Geometry: final body of the model. Coordinates: model frame, mm. A direction names the side the tool comes from. Give positions to 0.01 mm unless a question says otherwise; leave off trailing zeros. Write each loop counter-clockwise with the first axis right and the second up, starting at its lowest first coordinate (ties: lowest second). Pieces come first, ordered by that corner, then holes. Notation, with made-up numbers: M 2.5,70 L 20.5,70 A25 cw 20.5,104 Z; hole C 78.25,-37 d6. An arc over 180 degrees is marked long. Answer as a JSON object with one key per item and string values.
from build123d import *
from build123d.topology import SkipClean

# Parameters (mm, degrees)
SKETCH_1_R          = 3.25
EXTRUDE_1_DEPTH     = 29
CUT_EXTRUDE_START   = -5
SKETCH_2_OUTSIDE_W  = 14.584
SKETCH_2_OUTSIDE_H  = 14.584
SKETCH_2_OUTSIDE_R  = 2.25
CUT_EXTRUDE_1_DEPTH = 4.6
CHAMFER_1_SIZE      = 2.2
CHAMFER_1_SIZE2     = 1.270170592
SKETCH_3_R          = 5.3
EXTRUDE_2_DEPTH     = 2
EXTRUDE_3_DEPTH     = 13
CUT_EXTRUDE_START_2 = -4.2
CUT_EXTRUDE_2_DEPTH = 2.2
SKETCH_6_OUTSIDE_W  = 21.896
SKETCH_6_OUTSIDE_H  = 21.896
SKETCH_6_OUTSIDE_R  = 3.05
CUT_EXTRUDE_3_DEPTH = 2


with BuildPart() as part:
    # Эскиз1 → Бобышка-Вытянуть1 (new body)
    with BuildSketch(Plane(origin=(0, 0, 0), x_dir=(1, 0, 0), z_dir=(0, 1, 0))):
        with Locations(Location((0, 0, 0), (0, 0, 90))):
            Circle(SKETCH_1_R)
    extrude(amount=EXTRUDE_1_DEPTH)

    # Эскиз2 outside → Вырез-Вытянуть1 (cut)
    with BuildSketch(Plane(origin=(0, 29, 0), x_dir=(1, 0, 0), z_dir=(0, 1, 0)).offset(CUT_EXTRUDE_START)):
        Rectangle(SKETCH_2_OUTSIDE_W, SKETCH_2_OUTSIDE_H)
        with Locations(Location((0, 0, 0), (0, 0, 270))):
            Circle(SKETCH_2_OUTSIDE_R, mode=Mode.SUBTRACT)
    extrude(amount=-CUT_EXTRUDE_1_DEPTH, mode=Mode.SUBTRACT)

    # Фаска1
    chamfer_1_edges = [part.edges().sort_by_distance(p)[0] for p in [
        (0, 29, 3.25),
    ]]
    chamfer_1_side = [part.faces().sort_by_distance(p)[0] for p in [
        (0, 26.5, 3.25),
    ]]
    chamfer(chamfer_1_edges, length=CHAMFER_1_SIZE, length2=CHAMFER_1_SIZE2, reference=chamfer_1_side[0])

    # Эскиз3 → Бобышка-Вытянуть2 (add)
    with BuildSketch(Plane.XZ):
        with Locations(Location((0, 0, 0), (0, 0, 270))):
            Circle(SKETCH_3_R)
    extrude(amount=EXTRUDE_2_DEPTH)

    # Эскиз4 → Бобышка-Вытянуть3 (add)
    with BuildSketch(Plane.XZ.offset(2)):
        with BuildLine():
            Line((-0.65, 3.25), (0.65, 3.25))
            Line((0.65, 3.25), (0.65, 2.979932885))
            ThreePointArc((0.65, 2.979932885), (2.156675683, 2.156675683), (2.979932885, 0.65))
            Line((2.979932885, 0.65), (3.25, 0.65))
            Line((3.25, 0.65), (3.25, -0.65))
            Line((3.25, -0.65), (2.979932885, -0.65))
            ThreePointArc((2.979932885, -0.65), (2.156675683, -2.156675683), (0.65, -2.979932885))
            Line((0.65, -2.979932885), (0.65, -3.25))
            Line((0.65, -3.25), (-0.65, -3.25))
            Line((-0.65, -3.25), (-0.65, -2.979932885))
            ThreePointArc((-0.65, -2.979932885), (-2.156675683, -2.156675683), (-2.979932885, -0.65))
            Line((-2.979932885, -0.65), (-3.25, -0.65))
            Line((-3.25, -0.65), (-3.25, 0.65))
            Line((-3.25, 0.65), (-2.979932885, 0.65))
            ThreePointArc((-2.979932885, 0.65), (-2.156675683, 2.156675683), (-0.65, 2.979932885))
            Line((-0.65, 2.979932885), (-0.65, 3.25))
        make_face()
    extrude(amount=EXTRUDE_3_DEPTH)

    # Эскиз5 → Вырез-Вытянуть2 (cut)
    with BuildSketch(Plane.XZ.offset(15).offset(CUT_EXTRUDE_START_2)):
        with BuildLine():
            Line((-2.979932885, 0.65), (-1.94422221, 0.65))
            ThreePointArc((-1.94422221, 0.65), (-1.449568901, 1.449568901), (-0.65, 1.94422221))
            Line((-0.65, 1.94422221), (-0.65, 2.979932885))
            ThreePointArc((-0.65, 2.979932885), (-2.156675683, 2.156675683), (-2.979932885, 0.65))
        make_face()
        with BuildLine():
            Line((2.979932885, 0.65), (1.94422221, 0.65))
            ThreePointArc((1.94422221, 0.65), (1.449568901, 1.449568901), (0.65, 1.94422221))
            Line((0.65, 1.94422221), (0.65, 2.979932885))
            ThreePointArc((0.65, 2.979932885), (2.156675683, 2.156675683), (2.979932885, 0.65))
        make_face()
        with BuildLine():
            Line((-0.65, -1.94422221), (-0.65, -2.979932885))
            ThreePointArc((-0.65, -2.979932885), (-2.156675683, -2.156675683), (-2.979932885, -0.65))
            Line((-2.979932885, -0.65), (-1.94422221, -0.65))
            ThreePointArc((-1.94422221, -0.65), (-1.449568901, -1.449568901), (-0.65, -1.94422221))
        make_face()
        with BuildLine():
            Line((0.65, -2.979932885), (0.65, -1.94422221))
            ThreePointArc((0.65, -1.94422221), (1.449568901, -1.449568901), (1.94422221, -0.65))
            Line((1.94422221, -0.65), (2.979932885, -0.65))
            ThreePointArc((2.979932885, -0.65), (2.156675683, -2.156675683), (0.65, -2.979932885))
        make_face()
    extrude(amount=CUT_EXTRUDE_2_DEPTH, mode=Mode.SUBTRACT)

    # Эскиз6 outside → Вырез-Вытянуть3 (cut)
    with SkipClean():  # the faces are left unmerged after this step: merging them gives an invalid solid
        with BuildSketch(Plane.XZ.offset(15)):
            Rectangle(SKETCH_6_OUTSIDE_W, SKETCH_6_OUTSIDE_H)
            with Locations(Location((0, 0, 0), (0, 0, 102.304947534))):
                Circle(SKETCH_6_OUTSIDE_R, mode=Mode.SUBTRACT)
        extrude(amount=-CUT_EXTRUDE_3_DEPTH, mode=Mode.SUBTRACT)


solid = part.part
1) Set-up query: faces 1 (the cylindrical face through (1.4, -11.9, -1.5)), 2 (the flat face through (0.1, 0, -3.5)), 3 (the cylindrical face through (-1.5, -11.9, -1.4)), 4 (the flat face through (0.65, -11, 3)), 5 (the flat face through (-0.65, -11, 3)). Return all of +Z, -Z, +X, -X, +Y, -Y with unobstructed straight access to the full face (end or side cutting, diameter ignored); none if empty.
Geometry check:
{"face 1": "-Z, +X", "face 2": "+Y", "face 3": "-Z, -X", "face 4": "+Z, +X", "face 5": "+Z, -X"}
2) Cut plane B-B on x = 0. Return loops of the section in (y, z), and give its area (3 significant figures).
Geometry check:
{"outline": "M -15,-3.05 L -13,-3.05 L -13,-3.25 L -2,-3.25 L -2,-5.3 L 0,-5.3 L 0,-3.25 L 19.4,-3.25 L 19.4,-2.25 L 24,-2.25 L 24,-3.25 L 26.8,-3.25 L 29,-1.98 L 29,1.98 L 26.8,3.25 L 24,3.25 L 24,2.25 L 19.4,2.25 L 19.4,3.25 L 0,3.25 L 0,5.3 L -2,5.3 L -2,3.25 L -13,3.25 L -13,3.05 L -15,3.05 Z", "area": "281 mm2"}
3) Cut plane A-A on z = 0. Return loops of the section in (x, y), and give its area (3 significant figures).
Geometry check:
{"outline": "M -5.3,-2 L -3.25,-2 L -3.25,-13 L -3.05,-13 L -3.05,-15 L 3.05,-15 L 3.05,-13 L 3.25,-13 L 3.25,-2 L 5.3,-2 L 5.3,0 L 3.25,0 L 3.25,19.4 L 2.25,19.4 L 2.25,24 L 3.25,24 L 3.25,26.8 L 1.98,29 L -1.98,29 L -3.25,26.8 L -3.25,24 L -2.25,24 L -2.25,19.4 L -3.25,19.4 L -3.25,0 L -5.3,0 Z", "area": "281 mm2"}
4) Cut plane C-C on y = 5.5. Return loops of the section in (x, z).
Geometry check:
{"outline": "C 0,0 d6.5"}
5) Line query: line 1 (Y direction, x = -2, z = 1.5); line 2 (Z direction, x = 2, y = -11.5); line 3 (Y direction, x = -4.75, z = 2). Output: solid intervals per line, ascending. Write a range as from..to.
Geometry check:
{"line 1": "y = -15..-13, -10.8..19.4, 24..28.1", "line 2": "z = -0.65..0.65", "line 3": "y = -2..0"}
6) Cut plane D-D on x = -4.5. Return loops of the section in (y, z), and give its area (3 significant figures).
Geometry check:
{"outline": "M -2,-2.8 L 0,-2.8 L 0,2.8 L -2,2.8 Z", "area": "11.2 mm2"}
7) Contact query for flat-ended pins moving along their axis: P1, Ø5, axis at y = 24.5, z = 3, coming from the +X side; P2, Ø6, axis at x = -2.5, y = -10.5, coming from the +Z side; P3, Ø2, axis at y = -5.5, z = 0.5, coming from the -X side; P4, Ø1, axis at x = 3.5, y = 23, coming from the +Z side. Output: stop coordinate, or through.
Geometry check:
{"P1": "stops at x = 3.21", "P2": "stops at z = 3.25", "P3": "stops at x = -3.25", "P4": "passes through"}
8) Pull-direction query (Y, two-part tool) for faces 6 (the flat face through (0, 29, 0)), 7 (the cylindrical face through (2.139, -6.338, 2.174)), 8 (the flat face through (-2, -10.8, -2)); classes: pulls with the +Y half, pulls with the -Y half, needs draft (parallel to the pull), parting line crosses it, or undercut.
Geometry check:
{"face 6": "pulls with the +Y half", "face 7": "needs draft", "face 8": "undercut"}
